from build123d import *

# Parameters (mm, degrees)
F0_W     = 100
F0_H     = 914.4
F1_DEPTH = 100
F3_D     = 10
F4_D     = 10


with BuildPart() as f1:
    # F0 (on Top) → F1 (new body)
    with BuildSketch(Plane.XY):
        Polygon((0, 40), (0, 0), (214.8, 0), (214.8, -914.4), (0, -914.4), (0, -954.4), (609.6, -954.4), (609.6, -914.4), (394.8, -914.4), (394.8, 0), (609.6, 0), (609.6, 40), align=None)
        with Locations((304.8, -457.2)):
            Rectangle(F0_W, F0_H, mode=Mode.SUBTRACT)
    extrude(amount=F1_DEPTH)

    # F3 (through all)
    with Locations(Plane.YZ.offset(394.8)):
        with Locations((-40, 50)):
            Hole(F3_D / 2)

    # F4 (through all)
    with Locations(Plane.YZ.offset(394.8)):
        with Locations((-813.965738, 50)):
            Hole(F4_D / 2)


solid = f1.part
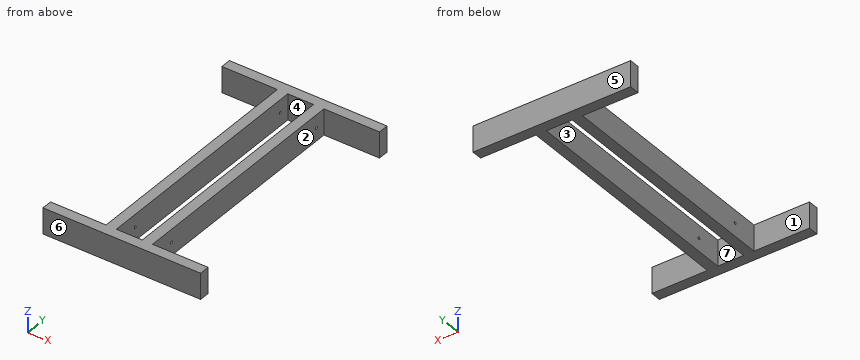
For this review, take the finished solid that the model builds, in its own axes (mm). Face numbers are marked on the shaded views. A direction names the side the tool comes from. Coordinates: 2 decimals unless noted, no trailing zeros. Order: outer loops, then holes, each group sorted by start corner. A loop starts at its lowest first (then second) coordinate and runs counter-clockwise, first axis right, second up. Notation, with made-up numbers: (71.25, 40) - (105.25, 40) arc R22 ccw to (105.25, 58) - close; hole circle Ø3 at (-10.5, 86.5). An arc over 180 degrees is marked (long way). Use one line per item in the form item = value.
Q1. Consider section A-A (x = 491.5). Give the boundary of the cut face in (y, z).
Checked values:
outline = (-954.4, 0) - (-914.4, 0) - (-914.4, 100) - (-954.4, 100) - close; (0, 0) - (40, 0) - (40, 100) - (0, 100) - close
Q2. Draft analysis for pull direction Y (two halves, no side actions). For the marked faces 4, 5, 6 and 7, state which applies: +Y half, -Y half, draft (parallel to the pull), parting line (faces both ways), or undercut.
Checked values:
face_4 = undercut
face_5 = +Y half
face_6 = -Y half
face_7 = undercut
Q3. For the marked faces 1, 2 and 3, list the 3-axis set-ups (+Z, -Z, +X, -X, +Y, -Y) from which the entire face can be reached by the end or side of a thin tool; tool diameter is ignored.
Checked values:
face_1 = +Z, -Z, -X
face_2 = +Z, -Z, +X
face_3 = +Z, -Z
Q4. Consider section B-B (z = 20). Give the boundary of the cut face in (x, y), then the cut area to 3 significant figures.
Checked values:
outline = (0, -954.4) - (609.6, -954.4) - (609.6, -914.4) - (394.8, -914.4) - (394.8, 0) - (609.6, 0) - (609.6, 40) - (0, 40) - (0, 0) - (214.8, 0) - (214.8, -914.4) - (0, -914.4) - close; hole (254.8, -914.4) - (354.8, -914.4) - (354.8, 0) - (254.8, 0) - close
area = 122,000 mm2
Q5. For P1, Ø3, axis at y = -549.5, z = 29.5, coming from the +X side; P2, Ø1.5, axis at y = -373, z = 20.5, coming from the -X side, all flat-tipped, find the tip position at first contact; note any pin that passes through.
Checked values:
P1 = 394.8
P2 = 214.8
Q6. For probe 1 along X at (y, z) = (-885, 15); probe 2 along Y at (x, z) = (214, 79), list the stretches that pass through material, from the lowest coordinate up. Write a range as from..to.
Checked values:
probe_1 = 214.8..254.8, 354.8..394.8
probe_2 = -954.4..-914.4, 0..40
Q7. Consider section C-C (y = -288). Give the boundary of the cut face in (x, z), then the cut area to 3 significant figures.
Checked values:
outline = (214.8, 0) - (254.8, 0) - (254.8, 100) - (214.8, 100) - close; (354.8, 0) - (394.8, 0) - (394.8, 100) - (354.8, 100) - close
area = 8,000 mm2
